Drawing for the job (mm, zero at the part's lowest x, y, z). A direction names the side the tool comes from. Give positions to 0.01 mm unless a question says otherwise; leave off trailing zeros. Loops run counter-clockwise (first coordinate to the right, second up) from the corner with the lowest first, then second, coordinate; pieces in that order, holes last. Notation, with made-up numbers: (-18.5, -34.5) - (19.5, -34.5) arc R22 cw to (19.5, -22.5) - close; hole circle Ø11 at (2, -11.5). An arc over 180 degrees is marked (long way). Return JSON: item names as keys, results as strings. Group by question number.
1) Drill centre lines: probe 1 along X at (y, z) = (19, 33); probe 2 along Z at (x, y) = (11, 30). Where is each one in solid material? Low to high. Write a range as from..to.
2) Mould opens along X. For the marked faces 1, 2 and 3 say: released by +X, released by -X, zero draft, split by the parting line, or undercut.
3) Slice it at C-C (z = 9). List the corners of the cut face in (x, y), and give its area (3 significant figures).
4) 3-axis set-ups, long thin cutter, end or side, ignore diameter. For the marked faces 4 and 5: which of +Z, -Z, +X, -X, +Y, -Y reach the whole face in a straight line?
5) Slice it at A-A (x = 19.05). List the corners of the cut face in (y, z).
6) Slice it at D-D (x = 10.5). List the corners of the cut face in (y, z).
7) Drop flat-ended pins along their axis: pin 1 (3 mm diameter, centred on y = 27, z = 54, fed in from -X); pin 2 (4 mm diameter, centred on y = 28.5, z = 63.5, fed in from -X); pin 3 (1.5 mm diameter, centred on y = 29.5, z = 42, fed in from -X). Give the stop position or say it passes through.
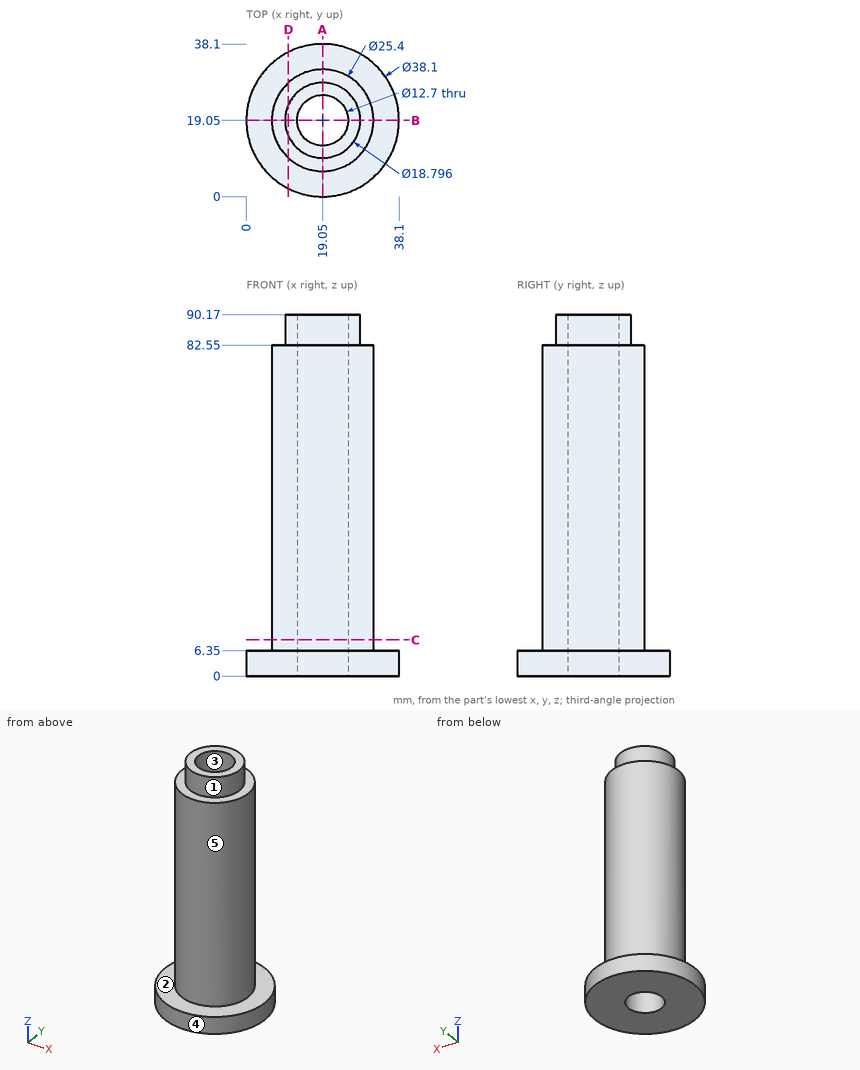
Results:
{
 "1": {"probe 1": "6.35..12.7, 25.4..31.75", "probe 2": "0..6.35"},
 "2": {"face 1": "split by the parting line", "face 2": "zero draft", "face 3": "undercut"},
 "3": {"outline": "circle Ø25.4 at (19.05, 19.05); hole circle Ø12.7 at (19.05, 19.05)", "area": "380 mm2"},
 "4": {"face 4": "+Z, -Z", "face 5": "+Z"},
 "5": {"outline": "(0, 0) - (12.7, 0) - (12.7, 90.17) - (9.65, 90.17) - (9.65, 82.55) - (6.35, 82.55) - (6.35, 6.35) - (0, 6.35) - close; (25.4, 0) - (38.1, 0) - (38.1, 6.35) - (31.75, 6.35) - (31.75, 82.55) - (28.45, 82.55) - (28.45, 90.17) - (25.4, 90.17) - close"},
 "6": {"outline": "(2.03, 0) - (36.07, 0) - (36.07, 6.35) - (28.44, 6.35) - (28.44, 82.55) - (22.95, 82.55) - (22.95, 90.17) - (15.15, 90.17) - (15.15, 82.55) - (9.66, 82.55) - (9.66, 6.35) - (2.03, 6.35) - close"},
 "7": {"pin 1": "x = 8.11", "pin 2": "x = 8.76", "pin 3": "x = 10.85"}
}
